Source: three-view drawing plus pictorial views. Frame: mm from the lowest corner of the part. A direction names the side the tool comes from. Round coordinates to 2 decimals unless told otherwise and drop trailing zeros. Loops run counter-clockwise (first coordinate to the right, second up) from the corner with the lowest first, then second, coordinate; pieces in that order, holes last. Notation, with made-up numbers: M -6.75,-22 L 34.25,-22 A30 ccw 34.25,7 Z; hole C -32,-14.5 d3. An arc over 180 degrees is marked long. Answer as a JSON object with one key per item and string values.
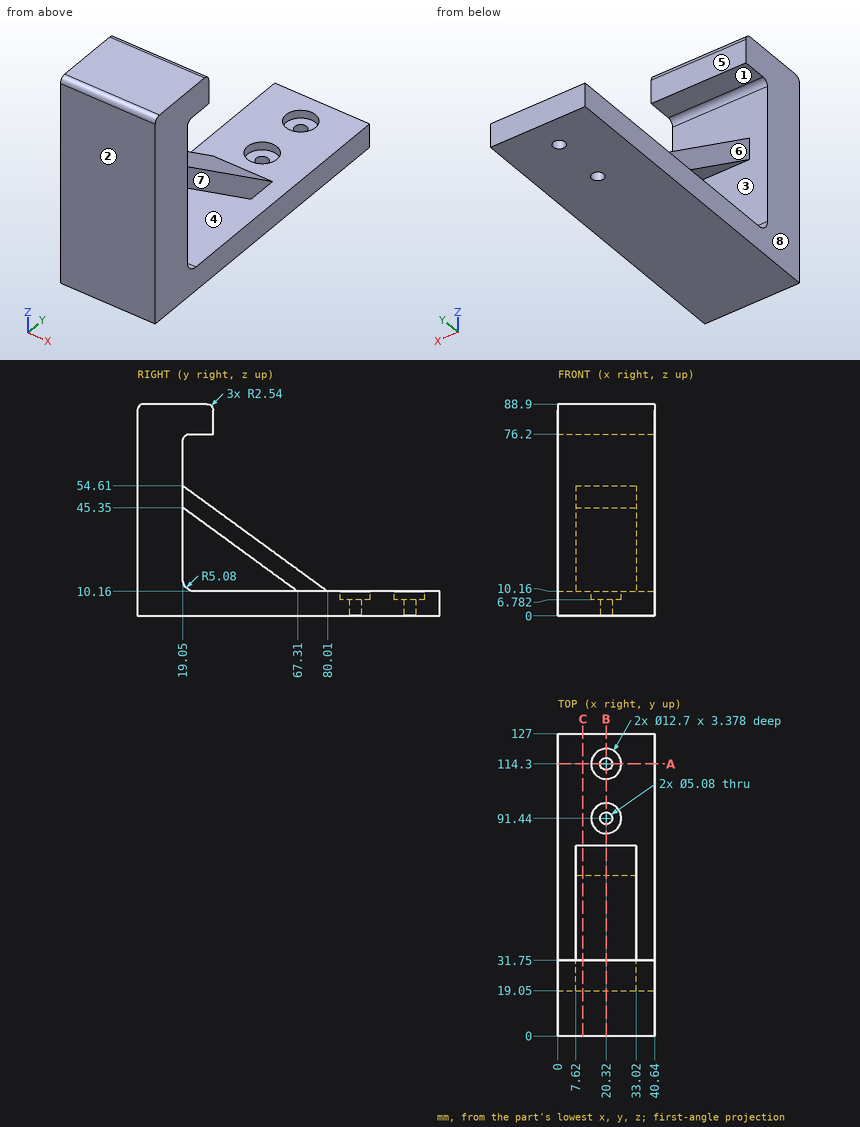
1) Cut plane C-C on x = 10.5. Return the cut outline in (y, z), and give its area (3 significant figures).
Geometry results:
{"outline": "M 0,0 L 127,0 L 127,10.16 L 80.01,10.16 L 19.05,54.61 L 19.05,73.66 A2.54 cw 21.59,76.2 L 31.75,76.2 L 31.75,86.36 A2.54 ccw 29.21,88.9 L 2.54,88.9 A2.54 ccw 0,86.36 Z; hole M 19.05,15.24 A5.08 ccw 24.13,10.16 L 67.31,10.16 L 19.05,45.35 Z", "area": "3,460 mm2"}
2) Cut plane A-A on y = 114.3. Return the cut outline in (x, z).
Geometry results:
{"outline": "M 0,0 L 17.78,0 L 17.78,6.78 L 13.97,6.78 L 13.97,10.16 L 0,10.16 Z; M 22.86,0 L 40.64,0 L 40.64,10.16 L 26.67,10.16 L 26.67,6.78 L 22.86,6.78 Z"}
3) Pull-direction query (Y, two-part tool) for the marked faces 1, 2, 3 and 4; classes: +Y half, -Y half, draft (parallel to the pull), parting line (faces both ways), or undercut.
Geometry results:
{"face 1": "draft", "face 2": "-Y half", "face 3": "undercut", "face 4": "undercut"}
4) First-contact query: pin 1 (10 mm diameter, centred on x = 20.32, y = 114.3, fed in from +Z); pin 2 (22 mm diameter, centred on y = 46, z = 32, fed in from -X); pin 3 (13.5 mm diameter, centred on y = 42, z = 40.5, fed in from +X); pin 4 (4 mm diameter, centred on x = 26.5, y = 64, fed in from -Z). Flat tips, straight axial feed; report the tip coordinate or a pass-through.
Geometry results:
{"pin 1": "z = 6.78", "pin 2": "x = 7.62", "pin 3": "x = 33.02", "pin 4": "z = 0"}
5) Set-up query: the marked faces 5, 6, 7 and 8. Return all of +Z, -Z, +X, -X, +Y, -Y with unobstructed straight access to the full face (end or side cutting, diameter ignored); none if empty.
Geometry results:
{"face 5": "+Z, +X, -X, +Y", "face 6": "-X, +Y", "face 7": "+X, +Y", "face 8": "+Z, -Z, -X, +Y, -Y"}
6) Line query: probe 1 along Y at (x, z) = (20.32, 4.25); probe 2 along Y at (x, z) = (20.32, 9.05); probe 3 along X at (y, z) = (114, 1). Output: solid intervals per line, ascending.
Geometry results:
{"probe 1": "0 to 88.9, 93.98 to 111.76, 116.84 to 127", "probe 2": "0 to 85.09, 97.79 to 107.95, 120.65 to 127", "probe 3": "0 to 17.8, 22.84 to 40.64"}
7) Cut plane B-B on x = 20.32. Count the separate pieces of the cut face and the enclosed holes in it, and give its area (3 significant figures).
Geometry results:
{"separate pieces": "3", "enclosed holes": "1", "area": "3,310 mm2"}
